Verification items for the finished model (mm, model axes). A direction names the side the tool comes from. Give positions to 0.01 mm unless a question says otherwise; leave off trailing zeros. Loops run counter-clockwise (first coordinate to the right, second up) from the corner with the lowest first, then second, coordinate; pieces in that order, holes last. Notation, with made-up numbers: (77.5, 55.5) -> (94.5, 55.5) arc R16 cw to (94.5, 85.5) -> close; hole circle Ø1 at (13, -29.75). An arc over 180 degrees is marked (long way). Answer in a Markdown table with one row per item. Add a question column.
Q1. Gauge pin test, flat ends, axial feed: P1, Ø6, axis at y = 8.5, z = -8.5, coming from the -X side; P2, Ø1, axis at x = -6, y = 22.5, coming from the -Z side; P3, Ø2, axis at y = 4.5, z = 5.5, coming from the +X side; P4, Ø6, axis at x = 0, z = 0, coming from the -Y side. Record the tip position at first contact, or that the pin passes through.
Q2. Section check D-D on x = 10.5. Enter the section's corners in (y, z).
Q3. Section check C-C on y = 10.5. Enter the section's corners in (x, z).
Q4. Material ranges on probe 1 along X at (y, z) = (15.75, 0); probe 2 along X at (y, z) = (24.5, 0), recorded low to high.
Q5. Section check A-A on x = 0. Enter the section's corners in (y, z), and give its area (3 significant figures).
Q6. Set-up check for faces 4 (the face through (-4.88, 25.07, -1.08)), 5 (the face through (4, 20, 4)): record each of +Z, -Z, +X, -X, +Y, -Y from which the full face is reachable in a straight line by a thin tool's end or side.
Q7. Release check for a two-part mould opening along Z. For faces 1 (the face through (6.513, 14.79, 16.243)), 2 (the face through (17, 0, -3)), 3 (the face through (16.855, 9.86, -2.213)) record: pulls with the +Z half, pulls with the -Z half, needs draft (parallel to the pull), parting line crosses it, or undercut.
Q8. Section check B-B on z = 0. Enter the section's corners in (x, y), and give its area (3 significant figures).
```python
from build123d import *

# Parameters (mm, degrees)
IZIM1_R                     = 17.5
IZIM1_R_2                   = 17
Y_KSEKLIK_EKSTR_ZYON1_DEPTH = 25
KAL_NLA_T_R2_START          = 20
KAL_NLA_T_R2_OUTLINE_R      = 17.5
KAL_NLA_T_R2_DEPTH          = 10
IZIM5_R                     = 5
KES_EKSTR_ZYON4_DEPTH       = 25


# Read off the part's stored shape, not the designer's step: Kalınlaştır2
with BuildPart() as part:
    # Çizim1 → Yükseklik-Ekstrüzyon1 (new body)
    with BuildSketch(Plane(origin=(0, 0, 0), x_dir=(1, 0, 0), z_dir=(0, 1, 0))):
        with Locations(Location((0, 0, 0), (0, 0, 270))):
            Circle(IZIM1_R)
        with Locations(Location((0, 0, 0), (0, 0, 270))):
            Circle(IZIM1_R_2, mode=Mode.SUBTRACT)
    extrude(amount=Y_KSEKLIK_EKSTR_ZYON1_DEPTH)

    # Kalınlaştır2 outline → Kalınlaştır2 (add)
    with BuildSketch(Plane(origin=(0, 0, 0), x_dir=(1, 0, 0), z_dir=(0, 1, 0)).offset(KAL_NLA_T_R2_START)):
        Circle(KAL_NLA_T_R2_OUTLINE_R)
    extrude(amount=KAL_NLA_T_R2_DEPTH)

    # Çizim5 → Kes-Ekstrüzyon4 (cut)
    with BuildSketch(Plane(origin=(0, 30, 0), x_dir=(1, 0, 0), z_dir=(0, 1, 0))):
        with Locations(Location((0, 0, 0), (0, 0, 270))):
            Circle(IZIM5_R)
    extrude(amount=-KES_EKSTR_ZYON4_DEPTH, mode=Mode.SUBTRACT)


solid = part.part
```
Taken from the geometry:
| question | item | result |
|---|---|---|
| 1 | P1 | stops at x = -16.61 |
| 1 | P2 | stops at z = -16.61 |
| 1 | P3 | stops at x = 16.91 |
| 1 | P4 | passes through |
| 2 | outline | (0, -14) -> (30, -14) -> (30, 14) -> (0, 14) -> (0, 13.37) -> (20, 13.37) -> (20, -13.37) -> (0, -13.37) -> close |
| 3 | outline | circle Ø35 at (0, 0); hole circle Ø34 at (0, 0) |
| 4 | probe 1 | x = -17.5 to -17, 17 to 17.5 |
| 4 | probe 2 | x = -17.5 to -5, 5 to 17.5 |
| 5 | outline | (0, -17.5) -> (30, -17.5) -> (30, -5) -> (20, -5) -> (20, -17) -> (0, -17) -> close; (0, 17) -> (20, 17) -> (20, 5) -> (30, 5) -> (30, 17.5) -> (0, 17.5) -> close |
| 5 | area | 270 mm² |
| 6 | face 4 | +Y, -Y |
| 6 | face 5 | -Y |
| 7 | face 1 | parting line crosses it |
| 7 | face 2 | needs draft |
| 7 | face 3 | undercut |
| 8 | outline | (-17.5, 0) -> (-17, 0) -> (-17, 20) -> (-5, 20) -> (-5, 30) -> (-17.5, 30) -> close; (5, 20) -> (17, 20) -> (17, 0) -> (17.5, 0) -> (17.5, 30) -> (5, 30) -> close |
| 8 | area | 270 mm² |
